Source: CAD feature listing. Evaluate the final solid. Frame: model axes, mm. A direction names the side the tool comes from. Give positions to 0.01 mm unless a question says otherwise; leave off trailing zeros. Loops run counter-clockwise (first coordinate to the right, second up) from the corner with the lowest first, then second, coordinate; pieces in that order, holes last. Notation, with made-up numbers: M -19.75,32.5 L 4.25,32.5 A20 ccw 4.25,55.5 Z; hole C 76.25,31 d9. An arc over 180 degrees is marked long. Put each result on its own line as item: value.
from build123d import *

# Parameters (mm, degrees)
BOSS_EXTRUDE1_DEPTH       = 8.13
F_3_0MM_DOWEL_HOLE1_D     = 3
F_3_0MM_DOWEL_HOLE1_DEPTH = 35
F_3_0MM_DOWEL_HOLE1_TIP   = 0.901290929
F_2_0MM_DOWEL_HOLE1_D     = 2
F_2_0MM_DOWEL_HOLE1_DEPTH = 35
F_2_0MM_DOWEL_HOLE1_TIP   = 0.600860619


with BuildPart() as part:
    # Sketch1 → Boss-Extrude1 (new body)
    with BuildSketch(Plane.XY):
        Polygon((-15.07, 0), (-15.07, 10.15), (-8.92, 10.15), (-8.92, 4.09), (8.92, 4.09), (8.92, 10.15), (15.07, 10.15), (15.07, 0), align=None)
    extrude(amount=BOSS_EXTRUDE1_DEPTH)

    # Ø3.0mm Dowel Hole1
    with Locations(Plane(origin=(0, 10.15, 0), x_dir=(1, 0, 0), z_dir=(0, 1, 0))):
        with Locations((-12.39, -4), (12.452, -4)):
            Hole(F_3_0MM_DOWEL_HOLE1_D / 2, depth=F_3_0MM_DOWEL_HOLE1_DEPTH)
            with Locations((0, 0, -(F_3_0MM_DOWEL_HOLE1_DEPTH + F_3_0MM_DOWEL_HOLE1_TIP / 2))):  # 118° drill point
                Cone(0, F_3_0MM_DOWEL_HOLE1_D / 2, F_3_0MM_DOWEL_HOLE1_TIP, mode=Mode.SUBTRACT)

    # Ø2.0mm Dowel Hole1
    with Locations(Plane(origin=(0, 4.09, 0), x_dir=(1, 0, 0), z_dir=(0, 1, 0))):
        with Locations((-6.53, -3.8), (6.53, -3.8)):
            Hole(F_2_0MM_DOWEL_HOLE1_D / 2, depth=F_2_0MM_DOWEL_HOLE1_DEPTH)
            with Locations((0, 0, -(F_2_0MM_DOWEL_HOLE1_DEPTH + F_2_0MM_DOWEL_HOLE1_TIP / 2))):  # 118° drill point
                Cone(0, F_2_0MM_DOWEL_HOLE1_D / 2, F_2_0MM_DOWEL_HOLE1_TIP, mode=Mode.SUBTRACT)


solid = part.part
1. Material intervals for line 1 (X direction, y = 7.5, z = 4); line 2 (X direction, y = 7, z = 1.5); line 3 (X direction, y = 5, z = 4.5), sorted ascending. Write a range as from..to.
Found:
line 1: -15.07..-13.89, -10.89..-8.92, 8.92..10.95, 13.95..15.07
line 2: -15.07..-8.92, 8.92..15.07
line 3: -15.07..-13.8, -10.98..-8.92, 8.92..11.04, 13.87..15.07
2. Section query B-B (x = -12.39). Output: boundary loops of the cut face in (y, z), plus the area to 3 significant figures.
Found:
outline: M 0,0 L 10.15,0 L 10.15,2.5 L 0,2.5 Z; M 0,5.5 L 10.15,5.5 L 10.15,8.13 L 0,8.13 Z
area: 52.1 mm^2
3. Section query C-C (x = 6.53). Output: boundary loops of the cut face in (y, z), plus the area to 3 significant figures.
Found:
outline: M 0,0 L 4.09,0 L 4.09,2.8 L 0,2.8 Z; M 0,4.8 L 4.09,4.8 L 4.09,8.13 L 0,8.13 Z
area: 25.1 mm^2
4. Contact query for flat-ended pins moving along their axis: P1, Ø2, axis at x = -7.5, z = 1, coming from the +Y side; P2, Ø2.5, axis at x = 12.452, z = 4, coming from the +Y side. Output: stop coordinate, or through.
Found:
P1: y = 4.09
P2: through
5. Draft query along X for faces 1 (the flat face through (-15.07, 5, 4)), 2 (the cylindrical face through (5.576, 2.016, 3.5)), 3 (the flat face through (0, 3, 8.13)). Return one class per face: pulls with the +X half, pulls with the -X half, needs draft (parallel to the pull), parting line crosses it, or undercut.
Found:
face 1: pulls with the -X half
face 2: undercut
face 3: needs draft
6. Access query for faces 4 (the flat face through (-8.92, 7, 4)), 5 (the flat face through (15.07, 5, 4)). Directions: +Z, -Z, +X, -X, +Y, -Y. A direction counts if a zero-diameter tool reaches every point of the face in a straight line with its end or side. Return the directions, or none.
Found:
face 4: +Z, -Z, +Y
face 5: +Z, -Z, +X, +Y, -Y
7. Section query A-A (y = 7.5). Output: boundary loops of the cut face in (x, z), plus the area to 3 significant figures.
Found:
outline: M -15.07,0 L -8.92,0 L -8.92,8.13 L -15.07,8.13 Z; M 8.92,0 L 15.07,0 L 15.07,8.13 L 8.92,8.13 Z; hole C -12.39,4 d3; hole C 12.45,4 d3
area: 85.9 mm^2
8. Section query D-D (z = 6). Output: boundary loops of the cut face in (x, y), plus the area to 3 significant figures.
Found:
outline: M -15.07,0 L 15.07,0 L 15.07,10.15 L 8.92,10.15 L 8.92,4.09 L -8.92,4.09 L -8.92,10.15 L -15.07,10.15 Z
area: 198 mm^2
